from build123d import *

# Parameters (mm, degrees)
SKETCH2_R          = 8.5725
EXTRUDE1_DEPTH     = 21.844
EXTRUDE1_TAPER     = -1.783333333
SKETCH5_OUTSIDE_W  = 73.012
SKETCH5_OUTSIDE_H  = 73.012
SKETCH5_OUTSIDE_R  = 7.528956448
CUT_EXTRUDE1_DEPTH = 22.8440001
CUT_EXTRUDE1_TAPER = 45
SKETCH8_R          = 14.9225
CUT_EXTRUDE4_DEPTH = 7.5532001
SKETCH9_OUTSIDE_W  = 26.06
SKETCH9_OUTSIDE_H  = 26.06
SKETCH9_OUTSIDE_R  = 7.655956448
CUT_EXTRUDE5_DEPTH = 1.058333333
SKETCH10_OUTSIDE_W = 56.444
SKETCH10_OUTSIDE_H = 56.444
SKETCH10_OUTSIDE_R = 7.655956448
CUT_EXTRUDE6_DEPTH = 15.232466767
CUT_EXTRUDE6_TAPER = 45
EXTRUDE2_DEPTH     = 6.5532
SKETCH7_OUTSIDE_W  = 107.462
SKETCH7_OUTSIDE_H  = 110.41
SKETCH7_OUTSIDE_R  = 9.525
CUT_EXTRUDE2_DEPTH = 22.8440001
CUT_EXTRUDE2_TAPER = 60
SKETCH18_OUTSIDE_W = 62.968
SKETCH18_OUTSIDE_H = 65.916
SKETCH18_OUTSIDE_R = 9.525
EXTRUDE3_DEPTH     = 10
EXTRUDE3_TAPER     = 60
SKETCH11_R         = 6.858
CUT_EXTRUDE7_DEPTH = 11.16
CUT_EXTRUDE7_TAPER = -1.783333333
SKETCH16_R         = 7.225132547
CUT_EXTRUDE9_DEPTH = 6.35
CUT_EXTRUDE9_TAPER = 45
SKETCH17_W         = 11.684
SKETCH17_H         = 6.399728224


with BuildPart() as part:
    # Sketch2 → Extrude1 (new body)
    with BuildSketch(Plane(origin=(-10.922, 0, 0), x_dir=(0, 0, -1), z_dir=(1, 0, 0))):
        Circle(SKETCH2_R)
    extrude(amount=EXTRUDE1_DEPTH, taper=EXTRUDE1_TAPER)

    # Sketch5 outside → Cut-Extrude1 (cut, through all)
    with BuildSketch(Plane(origin=(-10.922, 0, 0), x_dir=(0, 0, -1), z_dir=(1, 0, 0))):
        Rectangle(SKETCH5_OUTSIDE_W, SKETCH5_OUTSIDE_H)
        Circle(SKETCH5_OUTSIDE_R, mode=Mode.SUBTRACT)
    extrude(amount=CUT_EXTRUDE1_DEPTH, taper=CUT_EXTRUDE1_TAPER, mode=Mode.SUBTRACT)

    # Sketch8 → Cut-Extrude4 (cut, through all)
    with BuildSketch(Plane(origin=(4.3688, 0, 0), x_dir=(0, 0, -1), z_dir=(1, 0, 0))):
        Circle(SKETCH8_R)
    extrude(amount=CUT_EXTRUDE4_DEPTH, mode=Mode.SUBTRACT)

    # Sketch9 outside → Cut-Extrude5 (cut)
    with BuildSketch(Plane(origin=(4.3688, 0, 0), x_dir=(0, 0, -1), z_dir=(1, 0, 0))):
        Rectangle(SKETCH9_OUTSIDE_W, SKETCH9_OUTSIDE_H)
        Circle(SKETCH9_OUTSIDE_R, mode=Mode.SUBTRACT)
    extrude(amount=-CUT_EXTRUDE5_DEPTH, mode=Mode.SUBTRACT)

    # Sketch10 outside → Cut-Extrude6 (cut, through all)
    with BuildSketch(Plane(origin=(3.310466667, 0, 0), x_dir=(0, 0, -1), z_dir=(1, 0, 0))):
        Rectangle(SKETCH10_OUTSIDE_W, SKETCH10_OUTSIDE_H)
        Circle(SKETCH10_OUTSIDE_R, mode=Mode.SUBTRACT)
    extrude(amount=-CUT_EXTRUDE6_DEPTH, taper=CUT_EXTRUDE6_TAPER, mode=Mode.SUBTRACT)

    # Sketch6 → Extrude2 (add)
    with BuildSketch(Plane(origin=(10.922, 0, 0), x_dir=(0, 0, -1), z_dir=(1, 0, 0))):
        Polygon((0, 10.998522628), (-9.525, 5.499261314), (-9.525, -5.499261314), (0, -10.998522628), (9.525, -5.499261314), (9.525, 5.499261314), align=None)
    extrude(amount=-EXTRUDE2_DEPTH)

    # Sketch7 outside → Cut-Extrude2 (cut, through all)
    with BuildSketch(Plane(origin=(10.922, 0, 0), x_dir=(0, 0, -1), z_dir=(1, 0, 0))):
        Rectangle(SKETCH7_OUTSIDE_W, SKETCH7_OUTSIDE_H)
        Circle(SKETCH7_OUTSIDE_R, mode=Mode.SUBTRACT)
    extrude(amount=-CUT_EXTRUDE2_DEPTH, taper=CUT_EXTRUDE2_TAPER, mode=Mode.SUBTRACT)

    # Sketch18 outside → Extrude3 (cut)
    with BuildSketch(Plane.ZY.offset(-4.3688)):
        Rectangle(SKETCH18_OUTSIDE_W, SKETCH18_OUTSIDE_H)
        Circle(SKETCH18_OUTSIDE_R, mode=Mode.SUBTRACT)
    extrude(amount=-EXTRUDE3_DEPTH, taper=EXTRUDE3_TAPER, mode=Mode.SUBTRACT)

    # Sketch11 → Cut-Extrude7 (cut, through all)
    with BuildSketch(Plane(origin=(0.762, 0, 0), x_dir=(0, 0, -1), z_dir=(1, 0, 0))):
        Circle(SKETCH11_R)
    extrude(amount=CUT_EXTRUDE7_DEPTH, taper=CUT_EXTRUDE7_TAPER, mode=Mode.SUBTRACT)

    # Sketch16 → Cut-Extrude9 (cut)
    with BuildSketch(Plane(origin=(10.922, 0, 0), x_dir=(0, 0, -1), z_dir=(1, 0, 0))):
        Circle(SKETCH16_R)
    extrude(amount=-CUT_EXTRUDE9_DEPTH, taper=CUT_EXTRUDE9_TAPER, mode=Mode.SUBTRACT)

    # Sketch17 → Cut-Revolve1 (revolve, cut)
    with BuildSketch(Plane.XY):
        with Locations((-5.08, 3.199864112)):
            Rectangle(SKETCH17_W, SKETCH17_H)
    revolve(axis=Axis((-10.922, 0, 0), (1, 0, 0)), mode=Mode.SUBTRACT)


solid = part.part
Design review of the part built by this model. Coordinates are the model's own, in mm. A direction names the side the tool comes from. Give positions to 0.01 mm unless a question says otherwise; leave off trailing zeros. Loops run counter-clockwise (first coordinate to the right, second up) from the corner with the lowest first, then second, coordinate; pieces in that order, holes last. Notation, with made-up numbers: (-38, 65.5) -> (13, 65.5) arc R19 cw to (13, 95.5) -> close; hole circle Ø11 at (74.5, 71.5). An arc over 180 degrees is marked (long way). One line per question, with ' | ' between items. Start each with the question number.
(1) For line 1 (X direction, y = 4, z = 5.5); line 2 (Z direction, x = 6.75, y = -6.25); line 3 (Z direction, x = -2.5, y = 0), list the stretches that pass through material, from the lowest coordinate up.
(2) We need section C-C (x = 4). State the section outline as (y, z) points, and give its area (3 significant figures).
(3) We need section A-A (x = 7). State the section outline as (y, z) points (3 decimals).
(4) Insertion check: P1, Ø1.5, axis at x = 2.5, z = 0, coming from the -Y side; P2, Ø5, axis at y = -7.5, z = -2, coming from the -X side; P3, Ø1.5, axis at x = 6, z = 4.5, coming from the +Y side; P4, Ø7, axis at y = 2.5, z = 1, coming from the +X side. Each pin has a flat end and moves straight along its axis. Give the tip position at first contact, or say it passes through.
(5) We need section B-B (x = -7.25). State the section outline as (y, z) points.
(6) For faces 1 (the face through (3.847, -2.932, -7.072)), 2 (the face through (8, 0, -9.525)), list the 3-axis set-ups (+Z, -Z, +X, -X, +Y, -Y) from which the entire face can be reached by the end or side of a thin tool; tool diameter is ignored.
The answers:
1) line 1: x = -10.92 to 0.76 | line 2: z = -8.22 to -3.25, 3.25 to 8.22 | line 3: z = -8.83 to -6.4, 6.4 to 8.83
2) outline: circle Ø15.31 at (0, 0); hole circle Ø13.92 at (0, 0) | area: 32.0 mm^2
3) outline: (-10.999, 0) -> (-5.499, -9.525) -> (5.499, -9.525) -> (10.999, 0) -> (5.499, 9.525) -> (-5.499, 9.525) -> close; hole circle Ø14.104 at (0, 0)
4) P1: stops at y = -8.97 | P2: stops at x = -10.92 | P3: stops at y = 8.83 | P4: passes through
5) outline: circle Ø17.37 at (0, 0); hole circle Ø12.8 at (0, 0)
6) face 1: none | face 2: -Z, +X, -X, +Y, -Y
